Verification items for the finished model (mm, model axes). Face numbers are marked on the shaded views. A direction names the side the tool comes from. Round coordinates to 2 decimals unless told otherwise and drop trailing zeros. Order: outer loops, then holes, each group sorted by start corner. A loop starts at its lowest first (then second) coordinate and runs counter-clockwise, first axis right, second up. Notation, with made-up numbers: M -1,78.5 L 27,78.5 A8 ccw 27,93.5 Z; hole C -5.75,46 d6. An arc over 180 degrees is marked long. Answer as a JSON object with one key per item and string values. Group by question number.
```python
from build123d import *
from build123d.topology import SkipClean

# Parameters (mm, degrees)
ESBO_O1_R                = 11
RESSALTO_EXTRUS_O1_DEPTH = 1.9
RESSALTO_EXTRUS_O3_DEPTH = 3
ESBO_O4_R                = 3.25
CORTE_EXTRUS_O2_DEPTH    = 84.230548987
ESBO_O5_R                = 4
CORTE_EXTRUS_O5_DEPTH    = 3.9
RESSALTO_EXTRUS_O4_START = 3.25
ESBO_O6_R                = 11
RESSALTO_EXTRUS_O4_DEPTH = 3.25
ESBO_O7_R                = 4
CORTE_EXTRUS_O6_DEPTH    = 5.25
ESBO_O8_R                = 3.25
CORTE_EXTRUS_O7_DEPTH    = 84.320926451


with BuildPart() as part:
    # Esboço1 → Ressalto-extrusão1 (new body)
    with BuildSketch(Plane.XY):
        with Locations((13.384187511, -8.427486956)):
            Circle(ESBO_O1_R)
    extrude(amount=-RESSALTO_EXTRUS_O1_DEPTH)

    # Esboço3 → Ressalto-extrusão3 (add)
    with SkipClean():  # the faces are left unmerged after this step: merging them gives an invalid solid
        with BuildSketch(Plane(origin=(0, 0, -1.9), x_dir=(-1, 0, 0), z_dir=(0, 0, -1))):
            with BuildLine():
                Line((-24.384187511, -8.427486956), (-24.384187511, -68.427486956))
                ThreePointArc((-24.384187511, -68.427486956), (-13.384187511, -79.427486956), (-2.384187511, -68.427486956))
                Line((-2.384187511, -68.427486956), (-2.384187511, -8.427486956))
                ThreePointArc((-2.384187511, -8.427486956), (-13.384187511, 2.572513044), (-24.384187511, -8.427486956))
            make_face()
        extrude(amount=RESSALTO_EXTRUS_O3_DEPTH)

    # Esboço4 → Corte-extrusão2 (cut, through all)
    with SkipClean():  # the faces are left unmerged after this step: merging them gives an invalid solid
        with BuildSketch(Plane(origin=(0, 0, -4.9), x_dir=(-1, 0, 0), z_dir=(0, 0, -1))):
            with Locations((-13.384187511, -8.427486956)):
                Circle(ESBO_O4_R)
        extrude(amount=-CORTE_EXTRUS_O2_DEPTH, mode=Mode.SUBTRACT)

    # Esboço5 → Corte-extrusão5 (cut)
    with SkipClean():  # the faces are left unmerged after this step: merging them gives an invalid solid
        with BuildSketch(Plane(origin=(0, 0, -4.9), x_dir=(-1, 0, 0), z_dir=(0, 0, -1))):
            with Locations((-13.384187511, -8.427486956)):
                Circle(ESBO_O5_R)
        extrude(amount=-CORTE_EXTRUS_O5_DEPTH, mode=Mode.SUBTRACT)

    # Esboço6 → Ressalto-extrusão4 (add)
    with SkipClean():  # the faces are left unmerged after this step: merging them gives an invalid solid
        with BuildSketch(Plane.XY.offset(-1.9).offset(RESSALTO_EXTRUS_O4_START)):
            with Locations((13.384187511, -68.427486956)):
                Circle(ESBO_O6_R)
        extrude(amount=-RESSALTO_EXTRUS_O4_DEPTH)

    # Esboço7 → Corte-extrusão6 (cut)
    with SkipClean():  # the faces are left unmerged after this step: merging them gives an invalid solid
        with BuildSketch(Plane(origin=(0, 0, -4.9), x_dir=(-1, 0, 0), z_dir=(0, 0, -1))):
            with Locations((-13.384187511, -68.427486956)):
                Circle(ESBO_O7_R)
        extrude(amount=-CORTE_EXTRUS_O6_DEPTH, mode=Mode.SUBTRACT)

    # Esboço8 → Corte-extrusão7 (cut, through all)
    with SkipClean():  # the faces are left unmerged after this step: merging them gives an invalid solid
        with BuildSketch(Plane(origin=(0, 0, -4.9), x_dir=(-1, 0, 0), z_dir=(0, 0, -1))):
            with Locations((-13.384187511, -68.427486956)):
                Circle(ESBO_O8_R)
        extrude(amount=-CORTE_EXTRUS_O7_DEPTH, mode=Mode.SUBTRACT)


solid = part.part
```
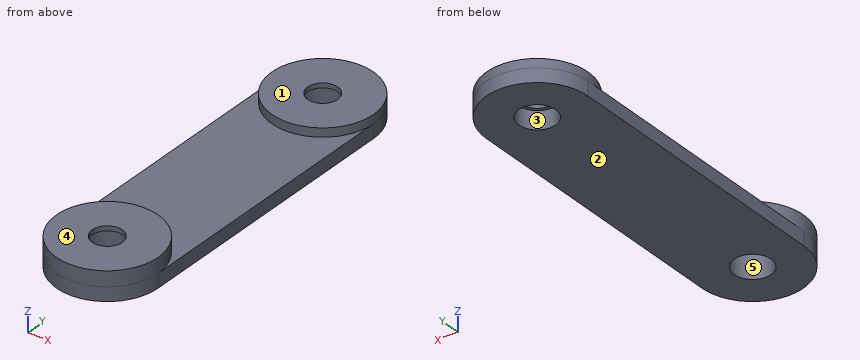
Q1. Thickness scan on line 1 (X direction, y = -68.5, z = -1.25); line 2 (Z direction, x = 7.5, y = -15.5); line 3 (Z direction, x = 20.5, y = -50.5). Record the ranges inside material, lowest first. Write a range as from..to.
Q2. Cross-section at C-C, the plane x = 20.75. Record the cut outline in (y, z), then the cut area to 3 significant figures.
Q3. Cross-section at A-A, the plane x = 13.75. Record the cut outline in (y, z), then the cut area to 3 significant figures.
Q4. Release check for a two-part mould opening along Y. For the marked faces 4 and 5 record: released by +Y, released by -Y, zero draft, split by the parting line, or undercut.
Q5. Gauge pin test, flat ends, axial feed: pin 1 Ø5 at (x, y) = (17, -18) entering from +Z; pin 2 Ø1 at (x, y) = (20.5, -36.5) entering from +Z; pin 3 Ø1 at (x, z) = (12.5, -2.5) entering from +Y. Record the tip position at first contact, or that the pin passes through.
Q6. Cross-section at B-B, the plane z = -3.5. Record the cut outline in (x, y).
Q7. Cross-section at D-D, the plane y = -36.5. Record the cut outline in (x, z).
Q8. Tool access check on the marked faces 1, 2 and 3. Record the directions out of +Z, -Z, +X, -X, +Y, -Y that give a thin tool (end or side, any length) a straight path to the whole face; none if there is none.
Conclusion:
{
 "1": {"line 1": "2.38..9.38, 17.38..24.38", "line 2": "-4.9..0", "line 3": "-4.9..-1.9"},
 "2": {"outline": "M -76.6,-4.9 L -0.26,-4.9 L -0.26,0 L -16.6,0 L -16.6,-1.9 L -60.26,-1.9 L -60.26,1.35 L -76.6,1.35 Z", "area": "313 mm2"},
 "3": {"outline": "M -79.42,-4.9 L -72.41,-4.9 L -72.41,0.35 L -71.66,0.35 L -71.66,1.35 L -79.42,1.35 Z; M -65.2,0.35 L -64.44,0.35 L -64.44,-4.9 L -12.41,-4.9 L -12.41,-1 L -11.66,-1 L -11.66,0 L -19.42,0 L -19.42,-1.9 L -57.43,-1.9 L -57.43,1.35 L -65.2,1.35 Z; M -5.2,-1 L -4.44,-1 L -4.44,-4.9 L 2.57,-4.9 L 2.57,0 L -5.2,0 Z", "area": "273 mm2"},
 "4": {"face 4": "zero draft", "face 5": "undercut"},
 "5": {"pin 1": "z = 0", "pin 2": "z = -1.9", "pin 3": "y = 2.57"},
 "6": {"outline": "M 2.38,-68.43 A11 ccw 24.38,-68.43 L 24.38,-8.43 A11 ccw 2.38,-8.43 Z; hole C 13.38,-68.43 d8; hole C 13.38,-8.43 d8"},
 "7": {"outline": "M 2.38,-4.9 L 24.38,-4.9 L 24.38,-1.9 L 2.38,-1.9 Z"},
 "8": {"face 1": "+Z, +X, -X, +Y", "face 2": "-Z, +X, -X, +Y, -Y", "face 3": "-Z"}
}
